Source: CAD feature listing. Evaluate the final solid. Frame: model axes, mm. A direction names the side the tool comes from. Give positions to 0.01 mm unless a question says otherwise; leave off trailing zeros. Order: outer loops, then holes, each group sorted by start corner. A loop starts at its lowest first (then second) coordinate and runs counter-clockwise, first axis right, second up. Notation, with made-up numbers: (-29, -37) - (24, -37) arc R25 ccw to (24, -20) - close; hole circle Ø10 at (67, -25). An arc over 180 degrees is marked (long way). Answer as CSV lines item,"result".
```python
from build123d import *

# Parameters (mm, degrees)
SKETCH_1_R           = 10.000000001
EXTRUDE_1_DEPTH      = 8
EXTRUDE_2_DEPTH      = 10
EXTRUDE_2_DEPTH_BACK = 18
EXTRUDE_4_DEPTH      = 20
EXTRUDE_4_TAPER      = 2
SKETCH_5_R           = 10
CUT_EXTRUDE_1_DEPTH  = 48
EXTRUDE_START        = -14
EXTRUDE_5_DEPTH      = 28
SKETCH_7_R           = 14
EXTRUDE_6_DEPTH      = 150
MOVE_BODY_1_ANGLE    = 160


# Read off the part's stored shape, not the designer's step: 凸台-拉伸3, 凸台-拉伸5
with BuildPart() as part:
    # 草图1 → 凸台-拉伸1 (new body)
    with BuildSketch(Plane.XY):
        Circle(SKETCH_1_R)
        with BuildLine():
            Line((-99.223415369, 15.875832346), (-71.057498037, 5.54717799))
            Line((-71.057498037, 5.54717799), (0, 0))
            Line((0, 0), (0, -25.00478934))
            Line((0, -25.00478934), (23.416407848, -26.832815739))
            add(Edge.make_bspline(
                [(23.416407848, -26.832815739), (23.559255777, -26.761391774), (23.857489252, -26.609782504), (24.343322546, -26.356143142), (25.001847908, -26.00202666), (25.895002872, -25.493833349), (26.689827796, -25.015527515), (27.443014709, -24.541367746), (28.44946677, -23.878396743), (30.180130615, -22.657518607), (32.463639395, -20.822910489), (35.803918719, -17.675778925), (39.356057937, -13.452382092), (43.810657679, -6.319948363), (47.26514501, 2.912424346), (48.687565133, 13.74600062), (47.956016905, 23.948129205), (45.527543401, 33.31383343), (41.766058602, 41.743075171), (35.35780408, 51.679214297), (25.341292826, 61.631560208), (11.525255636, 69.785622537), (-3.116720541, 74.453616351), (-17.875896804, 75.980775652), (-32.230785273, 74.726921151), (-50.32340393, 69.819482921), (-70.232141124, 58.486051284), (-85.364335796, 42.337960666), (-93.213462614, 29.471917912), (-96.911556554, 21.787367795), (-98.494293842, 17.864123943), (-99.223415369, 15.875832346)],
                knots=[0.039541182, 0.039541182, 0.039541182, 0.039541182, 0.040360106, 0.04117903, 0.042816878, 0.044454725, 0.046092573, 0.047730421, 0.049368269, 0.052643964, 0.059195355, 0.065746746, 0.078849528, 0.091952311, 0.118157875, 0.144363439, 0.170569003, 0.196774568, 0.222980132, 0.249185696, 0.301596825, 0.354007953, 0.406419082, 0.45883021, 0.511241339, 0.563652467, 0.668474724, 0.773296981, 0.82570811, 0.851913674, 0.878119238, 0.878119238, 0.878119238, 0.878119238], degree=3))
        make_face()
    extrude(amount=EXTRUDE_1_DEPTH)

    # 草图2 → 凸台-拉伸2 (add, two sides: drawn at the far end of the back side and taken through both)
    with BuildSketch(Plane(origin=(0, 0, 0), x_dir=(-1, 0, 0), z_dir=(0, 0, -1)).offset(-EXTRUDE_2_DEPTH_BACK)):
        with BuildLine():
            Line((-23.416407848, -26.832815739), (-18.944271899, -17.888543826))
            add(Edge.make_bspline(
                [(-18.944271899, -17.888543826), (-19.052705032, -17.834327259), (-19.279014375, -17.71924736), (-19.648152988, -17.526510294), (-20.157464576, -17.252862811), (-20.848872628, -16.859261983), (-21.642713236, -16.38143627), (-22.609327917, -15.759508594), (-24.135094314, -14.683161103), (-25.88889207, -13.274264185), (-28.481097704, -10.832666814), (-31.239689124, -7.553621002), (-34.737099736, -1.958117593), (-37.47574582, 5.346529302), (-38.623443824, 14.038278874), (-38.034234701, 22.314418593), (-35.383511893, 32.549710241), (-29.284340235, 43.56584113), (-19.178025873, 53.624814399), (-7.415995151, 60.576443845), (5.163786787, 64.593266285), (22.211265662, 66.362987302), (42.815452692, 62.532491918), (63.927151805, 50.528041572), (77.41272726, 36.156200275), (85.445738505, 22.987041434), (88.522694561, 16.010953304), (89.834776258, 12.432947561)],
                knots=[0.039541182, 0.039541182, 0.039541182, 0.039541182, 0.040360106, 0.04117903, 0.042816878, 0.044454725, 0.046092573, 0.049368269, 0.052643964, 0.059195355, 0.065746746, 0.078849528, 0.091952311, 0.118157875, 0.144363439, 0.170569003, 0.196774568, 0.249185696, 0.301596825, 0.354007953, 0.406419082, 0.45883021, 0.563652467, 0.668474724, 0.773296981, 0.82570811, 0.878119238, 0.878119238, 0.878119238, 0.878119238], degree=3))
            Line((89.834776258, 12.432947561), (99.223415369, 15.875832346))
            add(Edge.make_bspline(
                [(-23.416407848, -26.832815739), (-23.559255777, -26.761391774), (-23.857489252, -26.609782504), (-24.343322546, -26.356143142), (-25.001847908, -26.00202666), (-25.895002872, -25.493833349), (-26.689827796, -25.015527515), (-27.443014709, -24.541367746), (-28.44946677, -23.878396743), (-30.180130615, -22.657518607), (-32.463639395, -20.822910489), (-35.803918719, -17.675778925), (-39.356057937, -13.452382092), (-43.810657679, -6.319948363), (-47.26514501, 2.912424346), (-48.687565133, 13.74600062), (-47.956016905, 23.948129205), (-45.527543401, 33.31383343), (-41.766058602, 41.743075171), (-35.35780408, 51.679214297), (-25.341292826, 61.631560208), (-11.525255636, 69.785622537), (3.116720541, 74.453616351), (17.875896804, 75.980775652), (32.230785273, 74.726921151), (50.32340393, 69.819482921), (70.232141124, 58.486051284), (85.364335796, 42.337960666), (93.213462614, 29.471917912), (96.911556554, 21.787367795), (98.494293842, 17.864123943), (99.223415369, 15.875832346)],
                knots=[0.039541182, 0.039541182, 0.039541182, 0.039541182, 0.040360106, 0.04117903, 0.042816878, 0.044454725, 0.046092573, 0.047730421, 0.049368269, 0.052643964, 0.059195355, 0.065746746, 0.078849528, 0.091952311, 0.118157875, 0.144363439, 0.170569003, 0.196774568, 0.222980132, 0.249185696, 0.301596825, 0.354007953, 0.406419082, 0.45883021, 0.511241339, 0.563652467, 0.668474724, 0.773296981, 0.82570811, 0.851913674, 0.878119238, 0.878119238, 0.878119238, 0.878119238], degree=3))
        make_face()
    extrude(amount=EXTRUDE_2_DEPTH + EXTRUDE_2_DEPTH_BACK)

    # 凸台-拉伸3 outline → 凸台-拉伸3 (revolve)
    with BuildSketch(Plane.XZ):
        Polygon((10.000000001, 8), (10.000000001, 0), (0, 0), (0, -20), (24.306373953, -20), (25.004789342, 0), (24.725423186, 8), align=None)
    revolve(axis=Axis((0, 0, 0), (0, 0, 1)))

    # 草图4 → 凸台-拉伸4 (add)
    with BuildSketch(Plane.XY.offset(8)):
        with BuildLine():
            ThreePointArc((24.725423186, 0), (0.962911043, 24.706666187), (-24.650423647, 1.924361134))
            ThreePointArc((-24.650423647, 1.924361134), (-18.151132129, -16.789370273), (0, -24.725423186))
            ThreePointArc((0, -24.725423186), (17.483514403, -17.483514403), (24.725423186, 0))
        make_face()
    extrude(amount=EXTRUDE_4_DEPTH, taper=EXTRUDE_4_TAPER)

    # 草图5 → 切除-拉伸1 (cut)
    with BuildSketch(Plane(origin=(0, 0, -20), x_dir=(-1, 0, 0), z_dir=(0, 0, -1))):
        Circle(SKETCH_5_R)
    extrude(amount=-CUT_EXTRUDE_1_DEPTH, mode=Mode.SUBTRACT)

    # 凸台-拉伸5 outline → 凸台-拉伸5 (add)
    with BuildSketch(Plane.XY.offset(4).offset(EXTRUDE_START)):
        with BuildLine():
            Line((0, -42.050906086), (4.717060846, -47.040869425))
            Line((4.717060846, -47.040869425), (33.785028526, -19.562637042))
            Line((33.785028526, -19.562637042), (22.709671659, -7.846522593))
            ThreePointArc((22.709671659, -7.846522593), (13.94217781, -19.568157337), (0, -24.027007797))
            Line((0, -24.027007797), (0, -42.050906086))
        make_face()
    extrude(amount=EXTRUDE_5_DEPTH)

    # 草图7 → 凸台-拉伸6 (add)
    with BuildSketch(Plane(origin=(25.70930342, -27.19669848, 0), x_dir=(0, 0, -1), z_dir=(0.6869558095891056, -0.7266991920126075, 0))):
        with Locations((-4, -8.887114234)):
            Circle(SKETCH_7_R)
    extrude(amount=EXTRUDE_6_DEPTH)


with BuildPart() as part_1:
    # Move Body 1: moved
    add(part.part.rotate(Axis((0, 0, 0), (0, 0, -1)), MOVE_BODY_1_ANGLE))


solid = part_1.part
```
(1) Contact query for flat-ended pins moving along their axis: pin 1 (3 mm diameter, centred on x = 5, z = -1.5, fed in from +Y); pin 2 (10 mm diameter, centred on x = -111.5, z = -3.5, fed in from -Y); pin 3 (4 mm diameter, centred on x = -70, z = 11.5, fed in from +Y). Output: stop coordinate, or through.
Completed:
pin 1,"y = 24.71"
pin 2,"y = 48.97"
pin 3,"y = 59.82"
(2) Ray query, line 1 (X direction, y = 0, z = -9.5); line 2 (Z direction, x = -20.5, y = 18.5); line 3 (X direction, y = 0, z = 15.5). Return the intervals inside material, ascending. Write a range as from..to.
Completed:
line 1,"-41.18..-30.57, -24.81..-10, 10..24.67, 86.53..96.75"
line 2,"-10..18"
line 3,"-41.18..-30.57, -24.81..-10, 10..24.46, 86.53..96.75"
(3) Cut plane A-A (z = 21). Return loops of the section in (x, y), then the cut area to 3 significant figures.
Completed:
outline,"circle Ø48.54 at (0, 0); hole circle Ø20 at (0, 0)"
area,"1,540 mm²"
(4) Mould query, pull axis X, two halves, no side actions, for faces 1 (the flat face through (-163.68, 91.72, 4.2)), 2 (the flat face through (-22.947, 37.749, 3.804)), 3 (the flat face through (31, -58, 18)). Classes: released by +X, released by -X, zero draft, split by the parting line, or undercut.
Completed:
face 1,"released by -X"
face 2,"undercut"
face 3,"zero draft"
(5) Access query for faces 4 (the flat face through (46.56, 12.944, 3.944)), 5 (the flat face through (-4, 10, -20)), 6 (the flat face through (-26.97, 1.08, 12.93)), 7 (the cylindrical face through (-101.81, 45.42, 5.82)), 8 (the flat face through (31, -58, -10)). Directions: +Z, -Z, +X, -X, +Y, -Y. A direction counts if a zero-diameter tool reaches every point of the face in a straight line with its end or side. Return the directions, or none.
Completed:
face 4,"+Z, -Z, +Y"
face 5,"-Z, +X, -X, +Y, -Y"
face 6,"+Z"
face 7,"none"
face 8,"-Z"
